```python
from build123d import *

# Parameters (mm, degrees)
SKETCH1_R           = 1.1303
BOSS_EXTRUDE1_DEPTH = 6.35


with BuildPart() as part:
    # Sketch1 → Boss-Extrude1 (new body)
    with BuildSketch(Plane(origin=(0, 0, 0), x_dir=(1, 0, 0), z_dir=(0, 1, 0))):
        with BuildLine():
            Line((1.430315472, -2.155489974), (-22.62836127, -2.155489974))
            ThreePointArc((-22.62836127, -2.155489974), (-23.058725894, -2.096041852), (-23.456858243, -1.922149868))
            Line((-23.456858243, -1.922149868), (-37.881091448, 6.902829812))
            ThreePointArc((-37.881091448, 6.902829812), (-38.398503134, 7.18649116), (-38.959469005, 7.369510026))
            Line((-38.959469005, 7.369510026), (-75.77856814, 7.369510026))
            ThreePointArc((-75.77856814, 7.369510026), (-78.95356814, 4.194510026), (-75.77856814, 1.019510026))
            Line((-75.77856814, 1.019510026), (-51.211184528, 1.019510026))
            ThreePointArc((-51.211184528, 1.019510026), (-50.088652513, 0.554542041), (-49.623684528, -0.567989974))
            Line((-49.623684528, -0.567989974), (-49.623684528, -8.505489974))
            Line((-49.623684528, -8.505489974), (-47.083684528, -8.505489974))
            Line((-47.083684528, -8.505489974), (-47.083684528, -9.805489974))
            Line((-47.083684528, -9.805489974), (-48.988684528, -9.805489974))
            Line((-48.988684528, -9.805489974), (-48.988684528, -10.605489974))
            Line((-48.988684528, -10.605489974), (-40.48868451, -10.605489974))
            Line((-40.48868451, -10.605489974), (-40.48868451, -9.805489974))
            Line((-40.48868451, -9.805489974), (-42.39368451, -9.805489974))
            Line((-42.39368451, -9.805489974), (-42.39368451, -8.505489974))
            Line((-42.39368451, -8.505489974), (-39.85368451, -8.505489974))
            Line((-39.85368451, -8.505489974), (-39.85368451, -1.873214268))
            ThreePointArc((-39.85368451, -1.873214268), (-39.029938005, -0.481511409), (-37.413575094, -0.534105074))
            Line((-37.413575094, -0.534105074), (-25.626678473, -8.038809761))
            ThreePointArc((-25.626678473, -8.038809761), (-24.830413776, -8.386593729), (-23.969684528, -8.505489974))
            Line((-23.969684528, -8.505489974), (1.430315472, -8.505489974))
            ThreePointArc((1.430315472, -8.505489974), (4.605315472, -5.330489974), (1.430315472, -2.155489974))
        make_face()
        with Locations(Location((1.430315472, -5.330489974, 0), (0, 0, 270))):
            Circle(SKETCH1_R, mode=Mode.SUBTRACT)
    extrude(amount=BOSS_EXTRUDE1_DEPTH)


solid = part.part
```
Check sheet for the modelled part. Datum: model origin and axes. Units: mm. A direction names the side the tool comes from. Round coordinates to 2 decimals unless told otherwise and drop trailing zeros. Order: outer loops, then holes, each group sorted by start corner. A loop starts at its lowest first (then second) coordinate and runs counter-clockwise, first axis right, second up. Notation, with made-up numbers: (17.5, -24.75) -> (66.5, -24.75) arc R26 ccw to (66.5, 0.25) -> close; hole circle Ø11 at (-31, 84). An arc over 180 degrees is marked (long way). One line per item, written item: value. Start each with the question number.
Q1. Cross-section at C-C (x = -64). Record the boundary of the cut face in (y, z).
Q2. Set-up check for faces 4 (the face through (-38, 0, -1)), 5 (the face through (-10, 3, 2.155)), 6 (the face through (-42.394, 3, 9)), 7 (the face through (-31.603, 3.131, 4.234)), 8 (the face through (-48, 3, 9.805)): record each of +Z, -Z, +X, -X, +Y, -Y from which the full face is reachable in a straight line by a thin tool's end or side.
Q3. Gauge pin test, flat ends, axial feed: pin 1 Ø1 at (y, z) = (3, 5) entering from +X; pin 2 Ø1.9 at (x, y) = (-13, 4) entering from -Z; pin 3 Ø1.4 at (x, z) = (1.43, 5.33) entering from -Y; pin 4 Ø0.7 at (y, z) = (3.5, 9) entering from -X. Record the tip position at first contact, or that the pin passes through.
Q4. Thickness scan on line 1 (Z direction, x = -73, y = 2.75); line 2 (X direction, y = 3.25, z = 9.75); line 3 (Z direction, x = -9, y = 3.5). Record the ranges inside material, lowest first.
Q5. Cross-section at B-B (z = 5). Record the boundary of the cut face in (x, y).
Q6. Cross-section at D-D (x = -34). Record the boundary of the cut face in (y, z).
Q7. Mould release check, pull along Z, two halves, no side actions. Record for faces 1 (the face through (-64, 3, -1.02)), 2 (the face through (4.605, 3.131, 5.4)), 3 (the face through (-41, 3, 8.505)): pulls with the +Z half, pulls with the -Z half, needs draft (parallel to the pull), parting line crosses it, or undercut.
Completed:
1. outline: (0, -7.37) -> (6.35, -7.37) -> (6.35, -1.02) -> (0, -1.02) -> close
2. face 4: +Z, -Z, +X, -X, -Y
2. face 5: -Z, +X, +Y, -Y
2. face 6: +X, +Y, -Y
2. face 7: +Z, +Y, -Y
2. face 8: -X, +Y, -Y
3. pin 1: stops at x = 4.61
3. pin 2: stops at z = 2.16
3. pin 3: passes through
3. pin 4: stops at x = -47.08
4. line 1: z = -7.37 to -1.02
4. line 2: x = -47.08 to -42.39
4. line 3: z = 2.16 to 8.51
5. outline: (-49.62, 0) -> (-39.85, 0) -> (-39.85, 6.35) -> (-49.62, 6.35) -> close; (-30.4, 0) -> (0.35, 0) -> (0.35, 6.35) -> (-30.4, 6.35) -> close; (2.51, 0) -> (4.59, 0) -> (4.59, 6.35) -> (2.51, 6.35) -> close
6. outline: (0, -4.53) -> (6.35, -4.53) -> (6.35, 2.71) -> (0, 2.71) -> close
7. face 1: pulls with the +Z half
7. face 2: parting line crosses it
7. face 3: undercut
